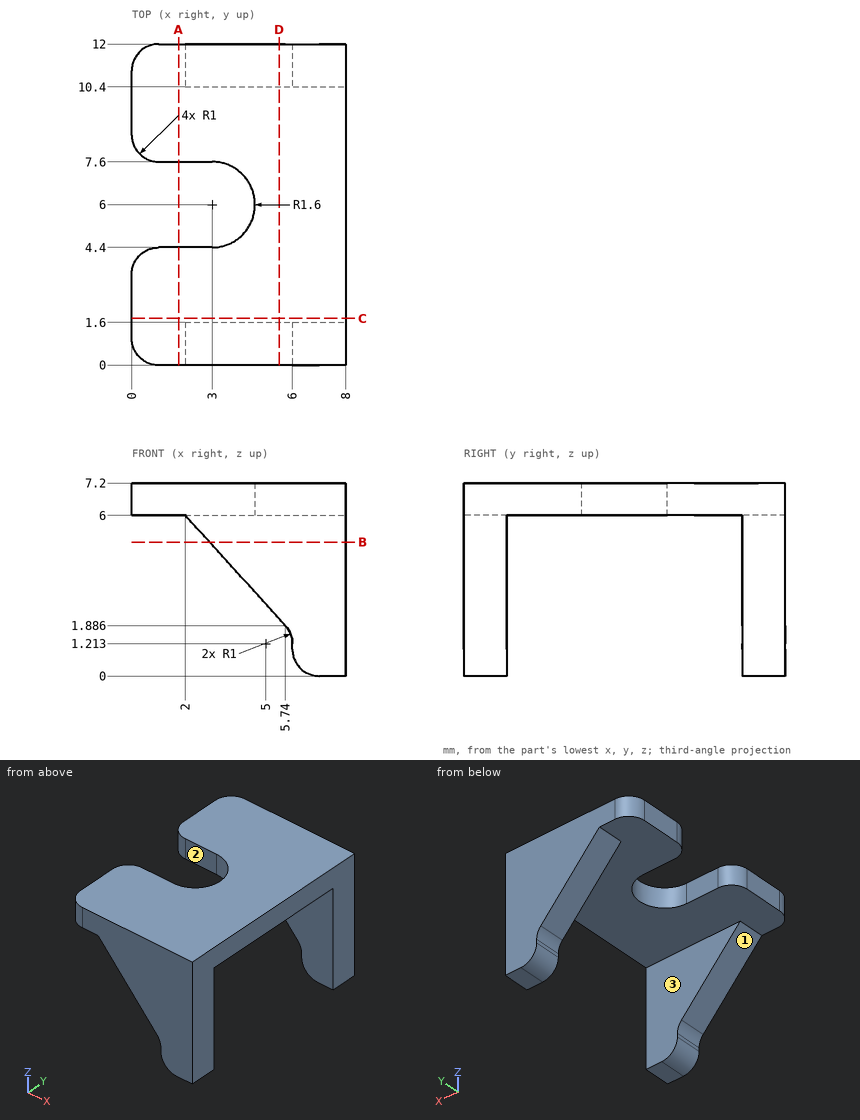
Job drawing, mm, ordinate dimensions from the low corner. One solid piece. A direction names the side the tool comes from. Round coordinates to 2 decimals unless told otherwise and drop trailing zeros. Loops run counter-clockwise (first coordinate to the right, second up) from the corner with the lowest first, then second, coordinate; pieces in that order, holes last. Notation, with made-up numbers: M 81.25,68 L 102.25,68 A28 ccw 102.25,103 Z; hole C -32,32 d9. An arc over 180 degrees is marked long. Answer as CSV lines item,"result".
1. Cut at C-C on y = 1.75. Write the cut outline in (x, z).
Resolved:
outline,"M 0,6 L 8,6 L 8,7.2 L 0,7.2 Z"
2. Cut at D-D on x = 5.5. Write the cut outline in (y, z).
Resolved:
outline,"M 0,2.15 L 1.6,2.15 L 1.6,6 L 10.4,6 L 10.4,2.15 L 12,2.15 L 12,7.2 L 0,7.2 Z"
3. 3-axis set-ups, long thin cutter, end or side, ignore diameter. For the marked faces 1, 2 and 3: which of +Z, -Z, +X, -X, +Y, -Y reach the whole face in a straight line?
Resolved:
face 1,"-Z, -X, +Y, -Y"
face 2,"+Z, -Z, -X"
face 3,"-Z, +X, -X"
4. Cut at B-B on z = 5. Write the cut outline in (x, y), then the cut area to 3 significant figures.
Resolved:
outline,"M 2.91,0 L 8,0 L 8,1.6 L 2.91,1.6 Z; M 2.91,10.4 L 8,10.4 L 8,12 L 2.91,12 Z"
area,"16.3 mm²"
5. Cut at A-A on x = 1.75. Write the cut outline in (y, z).
Resolved:
outline,"M 0,6 L 4.4,6 L 4.4,7.2 L 0,7.2 Z; M 7.6,6 L 12,6 L 12,7.2 L 7.6,7.2 Z"
6. Flat gauge pin, fed straight in: P1, Ø4, axis at x = 5.5, y = 7.5, coming from the -Z side. Where does the tip first touch, or does it go through?
Resolved:
P1,"stops at z = 6"
7. Wall check: probe 1 along Y at (x, z) = (3.5, 5.5); probe 2 along Y at (x, z) = (1.5, 6.25); probe 3 along Z at (x, y) = (6.5, 10). Give the ranges that are in metal, low to high. Write a range as [from, to].
Resolved:
probe 1,"y = [0, 1.6], [10.4, 12]"
probe 2,"y = [0, 4.4], [7.6, 12]"
probe 3,"z = [6, 7.2]"
